Source: three-view drawing plus pictorial views. Frame: mm from the lowest corner of the part. A direction names the side the tool comes from. Coordinates: 2 decimals unless noted, no trailing zeros. Loops run counter-clockwise (first coordinate to the right, second up) from the corner with the lowest first, then second, coordinate; pieces in that order, holes last. Notation, with made-up numbers: (69, 51) - (87, 51) arc R25 ccw to (87, 90) - close; hole circle Ø5 at (-0.75, 7.5). An arc over 180 degrees is marked (long way). Use CSV: the item, a comma, the result in double quotes. Start each with the question number.
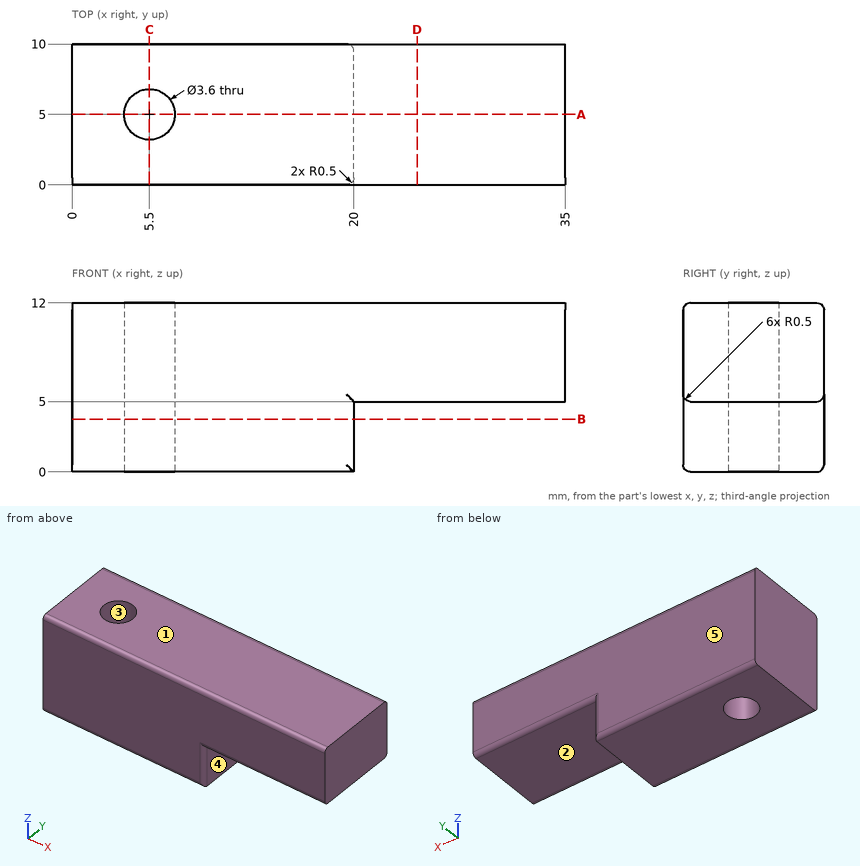
(1) Draft query along Y for the marked faces 3, 4 and 5. Return one class per face: released by +Y, released by -Y, zero draft, split by the parting line, or undercut.
(2) Reachability of the marked faces 1 and 2 from +Z, -Z, +X, -X, +Y, -Y: full face, straight path, thin tool, end or side. Return the list, or none.
(3) Section D-D on x = 24.5. Output: boundary loops of the cut face in (y, z), plus the area to 3 significant figures.
(4) Section B-B on z = 3.75. Output: boundary loops of the cut face in (x, y), plus the area to 3 significant figures.
(5) Pin query (flat end, axial travel): pin 1 Ø2.5 at (y, z) = (4.5, 2) entering from +X; pin 2 Ø4 at (x, z) = (23.5, 2.5) entering from -Y; pin 3 Ø2.5 at (x, y) = (28.5, 5.5) entering from -Z. Return the tip coordinate at first contact, or that it passes through.
(6) Section A-A on y = 5. Output: boundary loops of the cut face in (x, z).
(7) Ray query, line 1 (Y direction, x = 5.5, z = 9); line 2 (Z direction, x = 33.5, y = 4); line 3 (Y direction, x = 6, z = 1). Return the intervals inside material, ascending. Write a range as [from, to].
(8) Section C-C on x = 5.5. Output: boundary loops of the cut face in (y, z), plus the area to 3 significant figures.
Solution:
1,face 3,"undercut"
1,face 4,"zero draft"
1,face 5,"released by +Y"
2,face 1,"+Z, +X, -X, +Y, -Y"
2,face 2,"-Z, +X, +Y, -Y"
3,outline,"(0, 5.5) arc R0.5 ccw to (0.5, 5) - (9.5, 5) arc R0.5 ccw to (10, 5.5) - (10, 11.5) arc R0.5 ccw to (9.5, 12) - (0.5, 12) arc R0.5 ccw to (0, 11.5) - close"
3,area,"69.8 mm²"
4,outline,"(0, 0) - (19.5, 0) arc R0.5 ccw to (20, 0.5) - (20, 9.5) arc R0.5 ccw to (19.5, 10) - (0, 10) - close; hole circle Ø3.6 at (5.5, 5)"
4,area,"190 mm²"
5,pin 1,"stops at x = 20"
5,pin 2,"passes through"
5,pin 3,"stops at z = 5"
6,outline,"(0, 0) - (3.7, 0) - (3.7, 12) - (0, 12) - close; (7.3, 0) - (20, 0) - (20, 5) - (35, 5) - (35, 12) - (7.3, 12) - close"
7,line 1,"y = [0, 3.2], [6.8, 10]"
7,line 2,"z = [5, 12]"
7,line 3,"y = [0, 3.27], [6.73, 10]"
8,outline,"(0, 0.5) arc R0.5 ccw to (0.5, 0) - (3.2, 0) - (3.2, 12) - (0.5, 12) arc R0.5 ccw to (0, 11.5) - close; (6.8, 0) - (9.5, 0) arc R0.5 ccw to (10, 0.5) - (10, 11.5) arc R0.5 ccw to (9.5, 12) - (6.8, 12) - close"
8,area,"76.6 mm²"
